Check sheet for the modelled part. Datum: model origin and axes. Units: mm. A direction names the side the tool comes from. Round coordinates to 2 decimals unless told otherwise and drop trailing zeros. Write each loop counter-clockwise with the first axis right and the second up, starting at its lowest first coordinate (ties: lowest second). Pieces come first, ordered by that corner, then holes. Notation, with made-up numbers: M 31.25,45 L 90.25,45 A32 cw 90.25,81 Z; hole C 37,-20 d8. An arc over 180 degrees is marked long. Put each result on its own line as item: value.
```python
from build123d import *

# Parameters (mm, degrees)
SKETCH_1_R             = 6
EXTRUDE_1_DEPTH        = 150
HOLE_WIZARD_M6_1_D     = 5
HOLE_WIZARD_M6_1_DEPTH = 15
HOLE_WIZARD_M6_1_TIP   = 1.502151548
HOLE_WIZARD_M6_2_D     = 5
HOLE_WIZARD_M6_2_DEPTH = 15
HOLE_WIZARD_M6_2_TIP   = 1.502151548


with BuildPart() as part:
    # 草图1 → 凸台-拉伸1 (new, symmetric)
    with BuildSketch(Plane.XY):
        Circle(SKETCH_1_R)
    extrude(amount=EXTRUDE_1_DEPTH, both=True)

    # M6 螺纹孔1
    with Locations(Plane(origin=(0, 0, -150), x_dir=(-1, 0, 0), z_dir=(0, 0, -1))):
        with Locations((0, 0)):
            Hole(HOLE_WIZARD_M6_1_D / 2, depth=HOLE_WIZARD_M6_1_DEPTH)
            with Locations((0, 0, -(HOLE_WIZARD_M6_1_DEPTH + HOLE_WIZARD_M6_1_TIP / 2))):  # 118° drill point
                Cone(0, HOLE_WIZARD_M6_1_D / 2, HOLE_WIZARD_M6_1_TIP, mode=Mode.SUBTRACT)

    # M6 螺纹孔2
    with Locations(Plane.XY.offset(150)):
        with Locations((0, 0)):
            Hole(HOLE_WIZARD_M6_2_D / 2, depth=HOLE_WIZARD_M6_2_DEPTH)
            with Locations((0, 0, -(HOLE_WIZARD_M6_2_DEPTH + HOLE_WIZARD_M6_2_TIP / 2))):  # 118° drill point
                Cone(0, HOLE_WIZARD_M6_2_D / 2, HOLE_WIZARD_M6_2_TIP, mode=Mode.SUBTRACT)


solid = part.part
```
1. Cross-section at A-A (z = -95). Enter the section's corners in (x, y).
Computed values:
outline: C 0,0 d12
2. Depth check by flat-ended pin: pin 1 Ø3 at (x, z) = (3.5, 89.5) entering from -Y; pin 2 Ø1 at (x, y) = (-0.5, 1.5) entering from +Z; pin 3 Ø1 at (x, y) = (0.5, 0.5) entering from +Z. Enter the tip coordinate at first touch or a pass-through.
Computed values:
pin 1: stops at y = -5.66
pin 2: stops at z = 134.75
pin 3: stops at z = 134.22
3. Scan lines: probe 1 along Y at (x, z) = (0, -141.75); probe 2 along X at (y, z) = (-0.5, -125); probe 3 along X at (y, z) = (1.75, -9). Record each from-to range of solid material in increasing order.
Computed values:
probe 1: y = -6 to -2.5, 2.5 to 6
probe 2: x = -5.98 to 5.98
probe 3: x = -5.74 to 5.74
4. Release check for a two-part mould opening along Y. For faces 3 (the cylindrical face through (-6, 0, 2)), 4 (the conical face through (-0.094, -0.424, 133.759)), 5 (the flat face through (3, 0, -150)), 6 (the cylindrical face through (0.54, -2.44, 142.4)) record: +Y half, -Y half, draft (parallel to the pull), parting line (faces both ways), or undercut.
Computed values:
face 3: parting line
face 4: undercut
face 5: draft
face 6: undercut
5. Access from +Z, -Z, +X, -X, +Y, -Y to the whole of each face (thin tool, end or side, straight path). Record for faces 1 (the flat face through (3, 0, 150)), 2 (the cylindrical face through (-0.54, -2.44, -142.4)).
Computed values:
face 1: +Z, +X, -X, +Y, -Y
face 2: -Z
